```python
from build123d import *

# Parameters (mm, degrees)
BOSS_EXTRUDE1_DEPTH     = 10
BOSS_EXTRUDE2_START     = -10
BOSS_EXTRUDE2_DEPTH     = 76.2
SKETCH3_W               = 15
SKETCH3_H               = 22.225
REVOLVE1_ANGLE          = 300
CUT_EXTRUDE1_DEPTH      = 56
CUT_EXTRUDE1_DEPTH_BACK = 56
F_3_8_24_TAPPED_HOLE1_D = 8.4328


with BuildPart() as part:
    # Sketch1 → Boss-Extrude1 (new body)
    with BuildSketch(Plane(origin=(0, 0, 0), x_dir=(1, 0, 0), z_dir=(0, 1, 0))):
        with BuildLine():
            Line((15, 0), (15, 52.915026221))
            ThreePointArc((15, 52.915026221), (0, 55), (-15, 52.915026221))
            Line((-15, 52.915026221), (-15, 0))
            ThreePointArc((-15, 0), (0, -15), (15, 0))
        make_face()
    extrude(amount=BOSS_EXTRUDE1_DEPTH)

    # Sketch2 → Boss-Extrude2 (add)
    with BuildSketch(Plane(origin=(0, 10, 0), x_dir=(1, 0, 0), z_dir=(0, 1, 0)).offset(BOSS_EXTRUDE2_START)):
        with BuildLine():
            Line((-15, 26), (15, 26))
            Line((15, 26), (15, 52.915026221))
            ThreePointArc((15, 52.915026221), (0, 55), (-15, 52.915026221))
            Line((-15, 52.915026221), (-15, 26))
        make_face()
    extrude(amount=BOSS_EXTRUDE2_DEPTH)

    # Sketch3 → Revolve1 (revolve, symmetric)
    with BuildSketch(Plane(origin=(0, 0, 0), x_dir=(0, 0, -1), z_dir=(1, 0, 0))) as revolve1_sk:
        with Locations((47.5, 65.0875)):
            Rectangle(SKETCH3_W, SKETCH3_H)
    revolve(axis=Axis((0, 80.01, 0), (0, -1, 0)), revolution_arc=REVOLVE1_ANGLE / 2)
    revolve(revolve1_sk.sketch, axis=Axis((0, 80.01, 0), (0, 1, 0)), revolution_arc=REVOLVE1_ANGLE / 2)

    # Sketch4 → Cut-Extrude1 (cut, two sides)
    with BuildSketch(Plane(origin=(0, 0, 0), x_dir=(0, 0, -1), z_dir=(1, 0, 0))) as cut_extrude1_sk:
        Polygon((8, 53.975), (-17.734083046, 65.975), (-47.631397208, 65.975), (-47.631397208, 53.975), align=None)
    extrude(amount=CUT_EXTRUDE1_DEPTH, mode=Mode.SUBTRACT)
    extrude(cut_extrude1_sk.sketch, amount=-CUT_EXTRUDE1_DEPTH_BACK, mode=Mode.SUBTRACT)

    # 3/8-24 Tapped Hole1 (through all)
    with Locations(Plane(origin=(0, 10, 0), x_dir=(1, 0, 0), z_dir=(0, 1, 0))):
        with Locations((0, 0)):
            Hole(F_3_8_24_TAPPED_HOLE1_D / 2)


solid = part.part
```
Could you check a few things on this model? Use its own coordinates, in mm. A direction names the side the tool comes from. Coordinates: 2 decimals unless noted, no trailing zeros. Write each loop counter-clockwise with the first axis right and the second up, starting at its lowest first coordinate (ties: lowest second). Pieces come first, ordered by that corner, then holes. Notation, with made-up numbers: (26.5, 2.25) -> (31.5, 2.25) arc R26 cw to (31.5, 30.25) -> close; hole circle Ø7 at (10, 31). An arc over 180 degrees is marked (long way). Write item = value, one per line. Start each with the question number.
(1) I want a section at D-D (y = 64). Please give me the cut outline in (x, z).
(2) I want a section at B-B (z = -12.5). Please give me the cut outline in (x, y) (3 decimals).
(3) Will these pins go through, and if not, where does the flat tip stop? pin 1 (11 mm diameter, centred on x = 0, z = 0, fed in from -Y); pin 2 (9 mm diameter, centred on x = -1, y = 48.5, fed in from +Z); pin 3 (6 mm diameter, centred on x = -40, z = 30, fed in from -Y) (3 decimals); pin 4 (2 mm diameter, centred on x = 10.5, z = 8, fed in from +Y).
(4) I want a section at A-A (x = 0). Please give me the cut outline in (y, z).
(5) Which directions (+Z, -Z, +X, -X, +Y, -Y) give clear straight access to the entire face, cutting with the end or side of a thin tool? Please do faces 4 (the face through (-36, 65.975, 29)), 5 (the face through (-35, 53.975, -31)), 6 (the face through (15, 29, -32)), 7 (the face through (0, 43, -26)), 8 (the face through (-23.7, 71.16, 41.05)).
(6) We'd pull the mould along Z, two halves only. Please class faces 1 (the face through (36, 65.975, 29)), 2 (the face through (23.7, 71.16, 41.05)), 3 (the face through (-37.797, 67.713, -13.091)): released by +Z, released by -Z, zero draft, split by the parting line, or undercut.
(7) I need wall thicknesses on line 1 (Z direction, x = 0, y = 2.5); line 2 (Y direction, x = 37, z = 26.5) (3 decimals); line 3 (Y direction, x = -38, z = -38.5) (3 decimals). Which ranges of each line are inside material? Lowest first, please. Write a range as [from, to].
(8) I want a section at C-C (z = -40). Please give me the cut outline in (x, y) (3 decimals).
Result set:
q1.outline = (-53.32, 13.5) arc R55 ccw (long way) to (53.32, 13.5) -> (37.65, 13.5) arc R40 cw to (15, -37.08) -> (15, -26) -> (-15, -26) -> (-15, -37.08) arc R40 cw to (-37.65, 13.5) -> close
q2.outline = (-53.561, 53.975) -> (-37.997, 53.975) -> (-37.997, 76.2) -> (-53.561, 76.2) -> close; (-15, 0) -> (15, 0) -> (15, 10) -> (-15, 10) -> close; (37.997, 53.975) -> (53.561, 53.975) -> (53.561, 76.2) -> (37.997, 76.2) -> close
q3.pin_1 = 0
q3.pin_2 = -26
q3.pin_3 = 65.975
q3.pin_4 = 10
q4.outline = (0, -55) -> (76.2, -55) -> (76.2, -26) -> (10, -26) -> (10, -4.22) -> (0, -4.22) -> close; (0, 4.22) -> (10, 4.22) -> (10, 15) -> (0, 15) -> close
q5.face_4 = +Z, +X, -X, -Y
q5.face_5 = +Z, -Z, -X, -Y
q5.face_6 = +Z, -Y
q5.face_7 = +Z, +Y
q5.face_8 = +Z, +Y, -Y
q6.face_1 = zero draft
q6.face_2 = released by +Z
q6.face_3 = undercut
q7.line_1 = [-55, -4.22], [4.22, 15]
q7.line_2 = [65.975, 76.2]
q7.line_3 = [53.975, 76.2]
q8.outline = (-37.749, 53.975) -> (-15, 53.975) -> (-15, 0) -> (15, 0) -> (15, 53.975) -> (37.749, 53.975) -> (37.749, 76.2) -> (-37.749, 76.2) -> close
